CAD build for the part. Positions are in the model's coordinates, mm. Round coordinates to 2 decimals unless told otherwise and drop trailing zeros. Write each loop counter-clockwise with the first axis right and the second up, starting at its lowest first coordinate (ties: lowest second). Pieces come first, ordered by that corner, then holes. Notation, with made-up numbers: (-9.75, 33) - (8.25, 33) arc R6 ccw to (8.25, 37) - close; hole circle Ø7 at (72.5, 34.5). An arc over 180 degrees is marked (long way). Use one line per item in the form item = value. Start each with the question number.
Item 1: Pull direction Y, two halves, no side cores. Call faces 1 (the cylindrical face through (28.47, 8.96, 2.35)), 2 (the flat face through (-11.65, -8.56, 2.35)), 3 (the flat face through (-2, 2, 0)): +Y half, -Y half, draft (parallel to the pull), parting line (faces both ways), or undercut.
Item 2: Band-saw the part on D-D, the plane x = -12. List the corners of the cut face in (y, z), and give its area (3 significant figures).
Item 3: Band-saw the part on A-A, the plane y = 18. List the corners of the cut face in (x, z), and give its area (3 significant figures).
Item 4: Band-saw the part on B-B, the plane x = -22.5. List the corners of the cut face in (y, z).
Item 5: Drill centre lines: L1, parallel to X at y = 7.5, z = 2.6; L2, parallel to Y at x = 3, z = 1.35; L3, parallel to Y at x = -8, z = 3.4. Where is each one in solid material? Low to high.
Item 6: Band-saw the part on C-C, the plane z = 3.4. Give the number of separate pieces and of enclosed holes in the cut face, and give its area (3 significant figures).
Item 7: Pin check, flat tips, straight feed: pin 1 (2.5 mm diameter, centred on y = -4, z = 3.5, fed in from +X); pin 2 (0.5 mm diameter, centred on x = 1, z = 1.5, fed in from +Y); pin 3 (2 mm diameter, centred on x = -21.5, y = 22.5, fed in from +Z). Stop position of each tip, or through.
from build123d import *
from OCP.BRepAlgoAPI import BRepAlgoAPI_Cut
from OCP.TopTools import TopTools_ListOfShape

# Parameters (mm, degrees)
BOSS_EXTRUDE1_OUTLINE_R = 29.845
BOSS_EXTRUDE1_DEPTH     = 4.7625
FILLET1_R               = 6.35
CUT_EXTRUDE1_DEPTH      = 43.475049227


with BuildPart() as part:
    # Boss-Extrude1: read off the stored shape, not the designer's step
    # Boss-Extrude1 outline → Boss-Extrude1 (new body)
    with BuildSketch(Plane.XY):
        with Locations((2.773e-06, -3.1e-06)):
            Circle(BOSS_EXTRUDE1_OUTLINE_R)
        with BuildLine():
            Line((4.530888578, -4.449000046), (22.26219582, -14.686175534))
            ThreePointArc((22.26219582, -14.686175534), (-1.522e-06, -26.6700031), (-22.262195004, -14.686168364))
            Line((-22.262195004, -14.686168364), (-4.530889051, -4.448993916))
            ThreePointArc((-4.530889051, -4.448993916), (-1.522e-06, -6.3500031), (4.530888578, -4.449000046))
        make_face(mode=Mode.SUBTRACT)
        with BuildLine():
            Line((-6.11838599, -1.699361492), (-23.849694433, -11.936537069))
            ThreePointArc((-23.849694433, -11.936537069), (-23.096893005, 13.334999916), (-1.587497227, 26.622707951))
            Line((-1.587497227, 26.622707951), (-1.587497227, 6.148357962))
            ThreePointArc((-1.587497227, 6.148357962), (-5.499256774, 3.174999961), (-6.11838599, -1.699361492))
        make_face(mode=Mode.SUBTRACT)
        with BuildLine():
            Line((1.118068907, -0.999933056), (-1.118065826, -0.9999303))
            ThreePointArc((-1.118065826, -0.9999303), (4.622e-06, 1.499974165), (1.118068907, -0.999933056))
        make_face(mode=Mode.SUBTRACT)
        with BuildLine():
            Line((1.587502773, 6.148357962), (1.587502773, 26.622707951))
            ThreePointArc((1.587502773, 26.622707951), (23.096900555, 13.334996444), (23.849696391, -11.936544238))
            Line((23.849696391, -11.936544238), (6.118389237, -1.69936977))
            ThreePointArc((6.118389237, -1.69936977), (5.499264467, 3.17499624), (1.587502773, 6.148357962))
        make_face(mode=Mode.SUBTRACT)
    extrude(amount=BOSS_EXTRUDE1_DEPTH)

    # Fillet1
    fillet1_edges = [part.edges().sort_by_distance(p)[0] for p in [
        (4.530888578, -4.449000046, 2.38125),
        (-4.530889051, -4.448993916, 2.38125),
        (-22.262195004, -14.686168364, 2.38125),
        (22.26219582, -14.686175534, 2.38125),
        (-23.849694433, -11.936537069, 2.38125),
        (-6.11838599, -1.699361492, 2.38125),
        (-1.587497227, 6.148357962, 2.38125),
        (-1.587497227, 26.622707951, 2.38125),
        (1.587502773, 26.622707951, 2.38125),
        (1.587502773, 6.148357962, 2.38125),
        (6.118389237, -1.69936977, 2.38125),
        (23.849696391, -11.936544238, 2.38125),
    ]]
    fillet(fillet1_edges, radius=FILLET1_R)


with BuildPart() as cut_extrude1_tool:
    # Sketch2 → Cut-Extrude1 (new, through all)
    with BuildSketch(Plane.XY.offset(4.7625)):
        with BuildLine():
            Line((0.500000016, -0.999931678), (0, -0.999931678))
            Line((0, -0.999931678), (0, -6.3500031))
            ThreePointArc((0, -6.3500031), (0.250194284, -6.345072384), (0.500000016, -6.330287672))
            Line((0.500000016, -6.330287672), (0.500000016, -0.999931678))
        make_face()
        with BuildLine():
            Line((0, -6.3500031), (0, -0.999931678))
            Line((0, -0.999931678), (-0.500000016, -0.999931678))
            Line((-0.500000016, -0.999931678), (-0.500000016, -6.330287234))
            ThreePointArc((-0.500000016, -6.330287234), (-0.250194288, -6.345072165), (0, -6.3500031))
        make_face()
    extrude(amount=-CUT_EXTRUDE1_DEPTH)


with BuildPart() as part_1:
    add(part.part)

    # Cut-Extrude1: cut by cut_extrude1_tool, with a tolerance
    cut_extrude1_stock = TopTools_ListOfShape()
    cut_extrude1_stock.Append(part_1.part.wrapped)
    cut_extrude1_tools = TopTools_ListOfShape()
    cut_extrude1_tools.Append(cut_extrude1_tool.part.wrapped)
    cut_extrude1_cut = BRepAlgoAPI_Cut()
    cut_extrude1_cut.SetArguments(cut_extrude1_stock)
    cut_extrude1_cut.SetTools(cut_extrude1_tools)
    cut_extrude1_cut.SetFuzzyValue(0.00001)
    cut_extrude1_cut.Build()
    add(Compound.cast(cut_extrude1_cut.Shape()).solids(), mode=Mode.REPLACE)


solid = part_1.part
Determined:
q1.face_1 = parting line
q1.face_2 = undercut
q1.face_3 = draft
q2.outline = (-27.33, 0) - (-23.82, 0) - (-23.82, 4.76) - (-27.33, 4.76) - close; (-8.76, 0) - (-5.1, 0) - (-5.1, 4.76) - (-8.76, 4.76) - close; (23.82, 0) - (27.33, 0) - (27.33, 4.76) - (23.82, 4.76) - close
q2.area = 50.9 mm²
q3.outline = (-23.81, 0) - (-19.68, 0) - (-19.68, 4.76) - (-23.81, 4.76) - close; (-1.59, 0) - (1.59, 0) - (1.59, 4.76) - (-1.59, 4.76) - close; (19.68, 0) - (23.81, 0) - (23.81, 4.76) - (19.68, 4.76) - close
q3.area = 54.4 mm²
q4.outline = (-19.61, 0) - (-8.39, 0) - (-8.39, 4.76) - (-19.61, 4.76) - close; (14.32, 0) - (19.61, 0) - (19.61, 4.76) - (14.32, 4.76) - close
q5.L1 = -28.89 to -25.59, -2.06 to 2.06, 25.59 to 28.89
q5.L2 = -29.69 to -26.5, -5.69 to 5.92, 22.7 to 29.69
q5.L3 = -28.75 to -25.44, -6.45 to -2.51, 25.06 to 28.75
q6.separate_pieces = 1
q6.enclosed_holes = 3
q6.area = 981 mm²
q7.pin_1 = 29.72
q7.pin_2 = 29.84
q7.pin_3 = through
